from build123d import *

# Parameters (mm, degrees)
SKETCH_1_W                   = 50
SKETCH_1_H                   = 100
EXTRUDE_1_DEPTH              = 2
SKETCH_2_W                   = 3
SKETCH_2_H                   = 100
EXTRUDE_2_DEPTH              = 80
SKETCH_3_W                   = 2
SKETCH_3_H                   = 66.7
EXTRUDE_3_DEPTH              = 70
CUT_EXTRUDE_4_REACH          = 162.465
SKETCH_8_W                   = 2
SKETCH_8_H                   = 66.7
EXTRUDE_4_DEPTH              = 70
CUT_EXTRUDE_5_REACH          = 140.25
HOLE_WIZARD_M3_1_D           = 2.5
HOLE_WIZARD_M3_1_DEPTH       = 2
HOLE_WIZARD_M3_1_CSINK_D     = 3.05
HOLE_WIZARD_M3_1_CSINK_ANGLE = 90
FILLET_1_R                   = 2
CUT_EXTRUDE_6_REACH          = 140.25
SKETCH_12_R                  = 11
CUT_EXTRUDE_7_REACH          = 162.465
SKETCH_13_R                  = 14.5
SKETCH_14_W                  = 2
SKETCH_14_H                  = 66.7
EXTRUDE_5_DEPTH              = 70
CUT_EXTRUDE_8_REACH          = 156.14
SKETCH_15_R                  = 5.1
CUT_EXTRUDE_9_DEPTH          = 155.140358116
CUT_EXTRUDE_9_DEPTH_BACK     = 155.140358116
SKETCH_19_W                  = 2
SKETCH_19_H                  = 66.7
CUT_EXTRUDE_10_DEPTH         = 119.844436134
FILLET_2_R                   = 2
HOLE_WIZARD_M3_3_D           = 2.5
HOLE_WIZARD_M3_3_CSINK_D     = 3.05
HOLE_WIZARD_M3_3_CSINK_ANGLE = 90
CUT_EXTRUDE_11_DEPTH         = 134.88427839
CUT_EXTRUDE_11_DEPTH_BACK    = 134.88427839


# Read off the part's stored shape, not the designer's step: M1.6 螺纹孔1, M1.6 螺纹孔2, M2.5 螺纹孔1
with BuildPart() as part:
    # 草图1 → 凸台-拉伸1 (new body)
    with BuildSketch(Plane(origin=(0, 0, 0), x_dir=(1, 0, 0), z_dir=(0, 1, 0))):
        Rectangle(SKETCH_1_W, SKETCH_1_H)
    extrude(amount=EXTRUDE_1_DEPTH)

    # 草图2 → 凸台-拉伸2 (add)
    with BuildSketch(Plane(origin=(0, 2, 0), x_dir=(1, 0, 0), z_dir=(0, 1, 0))):
        with Locations((-23.5, 0)):
            Rectangle(SKETCH_2_W, SKETCH_2_H)
    extrude(amount=EXTRUDE_2_DEPTH)

    # 草图3 → 凸台-拉伸3 (add)
    with BuildSketch(Plane.ZY.offset(25)):
        with Locations((-49, 48.65)):
            Rectangle(SKETCH_3_W, SKETCH_3_H)
    extrude(amount=EXTRUDE_3_DEPTH)

    # 草图4 → 切除-拉伸4 (cut, up to next)
    with BuildSketch(Plane(origin=(0, 0, -50), x_dir=(-1, 0, 0), z_dir=(0, 0, -1)), mode=Mode.PRIVATE) as cut_extrude_4_sk1:
        with BuildLine():
            Line((95, 82), (61.65, 82))
            ThreePointArc((61.65, 82), (85.232011153, 72.232011153), (95, 48.65))
            Line((95, 48.65), (95, 82))
        make_face()
    cut_extrude_4_tool1 = extrude(cut_extrude_4_sk1.sketch, amount=-CUT_EXTRUDE_4_REACH, mode=Mode.PRIVATE) & part.part
    # 草图4 → 切除-拉伸4 (cut, up to next)
    with BuildSketch(Plane(origin=(0, 0, -50), x_dir=(-1, 0, 0), z_dir=(0, 0, -1)), mode=Mode.PRIVATE) as cut_extrude_4_sk2:
        with BuildLine():
            ThreePointArc((95, 48.65), (85.232011153, 25.067988847), (61.65, 15.3))
            Line((61.65, 15.3), (95, 15.3))
            Line((95, 15.3), (95, 48.65))
        make_face()
    cut_extrude_4_tool2 = extrude(cut_extrude_4_sk2.sketch, amount=-CUT_EXTRUDE_4_REACH, mode=Mode.PRIVATE) & part.part
    add(cut_extrude_4_tool1.solids().sort_by_distance((-87.550679, 74.550679, -50))[0], mode=Mode.SUBTRACT)
    add(cut_extrude_4_tool2.solids().sort_by_distance((-87.550679, 22.749321, -50))[0], mode=Mode.SUBTRACT)

    # 草图8 → 凸台-拉伸4 (add)
    with BuildSketch(Plane.ZY.offset(25)):
        with Locations((7, 48.65)):
            Rectangle(SKETCH_8_W, SKETCH_8_H)
    extrude(amount=EXTRUDE_4_DEPTH)

    # 草图9 → 切除-拉伸5 (cut, up to next)
    with BuildSketch(Plane.XY.offset(8), mode=Mode.PRIVATE) as cut_extrude_5_sk1:
        with BuildLine():
            ThreePointArc((-95, 48.65), (-85.232011153, 72.232011153), (-61.65, 82))
            Line((-61.65, 82), (-95, 82))
            Line((-95, 82), (-95, 48.65))
        make_face()
    cut_extrude_5_tool1 = extrude(cut_extrude_5_sk1.sketch, amount=-CUT_EXTRUDE_5_REACH, mode=Mode.PRIVATE) & part.part
    # 草图9 → 切除-拉伸5 (cut, up to next)
    with BuildSketch(Plane.XY.offset(8), mode=Mode.PRIVATE) as cut_extrude_5_sk2:
        with BuildLine():
            ThreePointArc((-61.65, 15.3), (-85.232011153, 25.067988847), (-95, 48.65))
            Line((-95, 48.65), (-95, 15.3))
            Line((-95, 15.3), (-61.65, 15.3))
        make_face()
    cut_extrude_5_tool2 = extrude(cut_extrude_5_sk2.sketch, amount=-CUT_EXTRUDE_5_REACH, mode=Mode.PRIVATE) & part.part
    add(cut_extrude_5_tool1.solids().sort_by_distance((-87.550679, 74.550679, 8))[0], mode=Mode.SUBTRACT)
    add(cut_extrude_5_tool2.solids().sort_by_distance((-87.550679, 22.749321, 8))[0], mode=Mode.SUBTRACT)

    # M3 螺纹孔1
    with Locations(Plane.XY.offset(8)):
        with Locations((-78.970508076, 38.65), (-61.65, 68.65), (-44.329491924, 38.65)):
            CounterSinkHole(HOLE_WIZARD_M3_1_D / 2, HOLE_WIZARD_M3_1_CSINK_D / 2, depth=HOLE_WIZARD_M3_1_DEPTH, counter_sink_angle=HOLE_WIZARD_M3_1_CSINK_ANGLE)

    # 圆角1
    fillet_1_edges = [part.edges().sort_by_distance(p)[0] for p in [
        (-23.5, 82, 50),
        (25, 1, 50),
        (25, 1, -50),
    ]]
    fillet(fillet_1_edges, radius=FILLET_1_R)

    # 草图12 → 切除-拉伸6 (cut, up to next)
    with BuildSketch(Plane.XY.offset(8), mode=Mode.PRIVATE) as cut_extrude_6_sk1:
        with Locations((-61.65, 48.65)):
            Circle(SKETCH_12_R)
    cut_extrude_6_tool1 = extrude(cut_extrude_6_sk1.sketch, amount=-CUT_EXTRUDE_6_REACH, mode=Mode.PRIVATE) & part.part
    add(cut_extrude_6_tool1.solids().sort_by_distance((-61.65, 48.65, 8))[0], mode=Mode.SUBTRACT)

    # 草图13 → 切除-拉伸7 (cut, up to next)
    with BuildSketch(Plane(origin=(0, 0, -50), x_dir=(-1, 0, 0), z_dir=(0, 0, -1)), mode=Mode.PRIVATE) as cut_extrude_7_sk1:
        with Locations((61.65, 48.65)):
            Circle(SKETCH_13_R)
    cut_extrude_7_tool1 = extrude(cut_extrude_7_sk1.sketch, amount=-CUT_EXTRUDE_7_REACH, mode=Mode.PRIVATE) & part.part
    add(cut_extrude_7_tool1.solids().sort_by_distance((-61.65, 48.65, -50))[0], mode=Mode.SUBTRACT)

    # 草图14 → 凸台-拉伸5 (add)
    with BuildSketch(Plane.ZY.offset(25)):
        with Locations((-38.5, 48.65)):
            Rectangle(SKETCH_14_W, SKETCH_14_H)
    extrude(amount=EXTRUDE_5_DEPTH)

    # 草图15 → 切除-拉伸8 (cut, up to next)
    with BuildSketch(Plane(origin=(0, 0, -39.5), x_dir=(-1, 0, 0), z_dir=(0, 0, -1)), mode=Mode.PRIVATE) as cut_extrude_8_sk1:
        with Locations(Location((61.65, 48.65, 0), (0, 0, 90))):
            Circle(SKETCH_15_R)
    cut_extrude_8_tool1 = extrude(cut_extrude_8_sk1.sketch, amount=-CUT_EXTRUDE_8_REACH, mode=Mode.PRIVATE) & part.part
    add(cut_extrude_8_tool1.solids().sort_by_distance((-61.65, 48.65, -39.5))[0], mode=Mode.SUBTRACT)

    # 草图18 → 切除-拉伸9 (cut, two sides: drawn at the far end of the back side and taken through both)
    with BuildSketch(Plane(origin=(0, 0, -39.5), x_dir=(-1, 0, 0), z_dir=(0, 0, -1)).offset(-CUT_EXTRUDE_9_DEPTH_BACK)):
        with BuildLine():
            Line((95, 15.3), (95, 48.65))
            ThreePointArc((95, 48.65), (85.232011153, 25.067988847), (61.65, 15.3))
            Line((61.65, 15.3), (95, 15.3))
        make_face()
        with BuildLine():
            Line((95, 48.65), (95, 82))
            Line((95, 82), (61.65, 82))
            ThreePointArc((61.65, 82), (85.232011153, 72.232011153), (95, 48.65))
        make_face()
    extrude(amount=CUT_EXTRUDE_9_DEPTH + CUT_EXTRUDE_9_DEPTH_BACK, mode=Mode.SUBTRACT)

    # 草图19 → 切除-拉伸10 (cut, through all)
    with BuildSketch(Plane.ZY.offset(25)):
        with Locations((-49, 48.65)):
            Rectangle(SKETCH_19_W, SKETCH_19_H)
    extrude(amount=CUT_EXTRUDE_10_DEPTH, mode=Mode.SUBTRACT)

    # 圆角2
    fillet_2_edges = [part.edges().sort_by_distance(p)[0] for p in [
        (-23.5, 82, -50),
    ]]
    fillet(fillet_2_edges, radius=FILLET_2_R)

    # M3 螺纹孔3 (through all)
    with Locations(Plane(origin=(0, 2, 0), x_dir=(1, 0, 0), z_dir=(0, 1, 0))):
        with Locations((-2.7, 0), (21, 10), (21, -10)):
            CounterSinkHole(HOLE_WIZARD_M3_3_D / 2, HOLE_WIZARD_M3_3_CSINK_D / 2, counter_sink_angle=HOLE_WIZARD_M3_3_CSINK_ANGLE)

    # M1.6 螺纹孔1 outline → M1.6 螺纹孔1 (revolve, cut)
    with BuildSketch(Plane(origin=(10, 0, -28), x_dir=(1, 0, 0), z_dir=(0, 0, 1))):
        Polygon((0, 0), (0.625, 0), (0.625, 1.8), (0.825, 2), (0, 2), align=None)
    revolve(axis=Axis((10, 0, -28), (0, 1, 0)), mode=Mode.SUBTRACT)

    # Hole Wizard M1.6 _1 2 outline → Hole Wizard M1.6 _1 2 (revolve, cut)
    with BuildSketch(Plane(origin=(6.4, 0, -28), x_dir=(1, 0, 0), z_dir=(0, 0, 1))):
        Polygon((0, 0), (0.625, 0), (0.625, 1.8), (0.825, 2), (0, 2), align=None)
    revolve(axis=Axis((6.4, 0, -28), (0, 1, 0)), mode=Mode.SUBTRACT)

    # M1.6 螺纹孔2 outline → M1.6 螺纹孔2 (revolve, cut)
    with BuildSketch(Plane(origin=(10, 0, -22), x_dir=(1, 0, 0), z_dir=(0, 0, 1))):
        Polygon((0, 0), (0.625, 0), (0.625, 1.8), (0.825, 2), (0, 2), align=None)
    revolve(axis=Axis((10, 0, -22), (0, 1, 0)), mode=Mode.SUBTRACT)

    # Hole Wizard M1.6 _2 2 outline → Hole Wizard M1.6 _2 2 (revolve, cut)
    with BuildSketch(Plane(origin=(6.4, 0, -22), x_dir=(1, 0, 0), z_dir=(0, 0, 1))):
        Polygon((0, 0), (0.625, 0), (0.625, 1.8), (0.825, 2), (0, 2), align=None)
    revolve(axis=Axis((6.4, 0, -22), (0, 1, 0)), mode=Mode.SUBTRACT)

    # 草图28 → 切除-拉伸11 (cut, two sides: drawn at the far end of the back side and taken through both)
    with BuildSketch(Plane(origin=(0, 2, 0), x_dir=(1, 0, 0), z_dir=(0, 1, 0)).offset(-CUT_EXTRUDE_11_DEPTH_BACK)):
        Polygon((-25, 37.5), (-95, 37.5), (-95, 39.5), (-25, 39.5), (-25, 50), (25, 50), (25, -50), (-25, -50), align=None)
    extrude(amount=CUT_EXTRUDE_11_DEPTH + CUT_EXTRUDE_11_DEPTH_BACK, mode=Mode.SUBTRACT)

    # M2.5 螺纹孔1 outline → M2.5 螺纹孔1 (revolve, cut)
    with BuildSketch(Plane(origin=(-29, 19, 0), x_dir=(1, 0, 0), z_dir=(0, -1, 0))):
        Polygon((0, 6), (1.025, 6), (1.025, 7.75), (1.275, 8), (0, 8), align=None)
    revolve(axis=Axis((-29, 19, 0), (0, 0, 1)), mode=Mode.SUBTRACT)

    # Hole Wizard M2.5 _1 2 outline → Hole Wizard M2.5 _1 2 (revolve, cut)
    with BuildSketch(Plane(origin=(-29, 27, 0), x_dir=(1, 0, 0), z_dir=(0, -1, 0))):
        Polygon((0, 6), (1.025, 6), (1.025, 7.75), (1.275, 8), (0, 8), align=None)
    revolve(axis=Axis((-29, 27, 0), (0, 0, 1)), mode=Mode.SUBTRACT)


solid = part.part
Build history of the part. All positions in model axes, mm. Round coordinates to 2 decimals unless told otherwise and drop trailing zeros. Loops run counter-clockwise (first coordinate to the right, second up) from the corner with the lowest first, then second, coordinate; pieces in that order, holes last. Notation, with made-up numbers: (51, 18) -> (61, 18) arc R12 cw to (61, 26) -> close; hole circle Ø4 at (0.5, 71). An arc over 180 degrees is marked (long way). One line per item, written item: value. Start each with the question number.
Q1. Probe line 1 along Y through (x, z) = (-61.65, 7); line 2 along Y through (x, z) = (-29, 6.8) (3 decimals); line 3 along X through (y, z) = (38.65, 6.75). List the from-to ranges inside material, lowest first.
Q2. Cut at A-A on z = 6.95. Count the separate pieces of the cut face and the enclosed holes in it, plus the area to 3 significant figures.
Q3. Cut at B-B on y = 27. List the corners of the cut face in (x, z) (3 decimals).
Q4. Two-plate mould, pull along Y, no slides. Class faces 1 (the face through (-52, 56, 8)), 2 (the face through (-43, 15.3, 7)), 3 (the face through (-45.001, 39.704, 6.85)): released by +Y, released by -Y, zero draft, split by the parting line, or undercut.
Q5. Cut at C-C on x = -68.5. List the corners of the cut face in (y, z), plus the area to 3 significant figures.
Computed:
1. line 1: 15.3 to 37.65, 59.65 to 67.4, 69.9 to 82
1. line 2: 15.3 to 17.975, 20.025 to 25.975, 28.025 to 82
1. line 3: -93.47 to -80.22, -77.72 to -66.23, -57.07 to -45.58, -43.08 to -25
2. separate pieces: 1
2. enclosed holes: 6
2. area: 3,790 mm²
3. outline: (-87.017, 6) -> (-30.025, 6) -> (-30.025, 7.75) -> (-30.275, 8) -> (-87.017, 8) -> close; (-27.975, 6) -> (-25, 6) -> (-25, 8) -> (-27.725, 8) -> (-27.975, 7.75) -> close
4. face 1: zero draft
4. face 2: released by -Y
4. face 3: undercut
5. outline: (16.01, 6) -> (40.04, 6) -> (40.04, 8) -> (16.01, 8) -> close; (57.26, 6) -> (81.29, 6) -> (81.29, 8) -> (57.26, 8) -> close
5. area: 96.1 mm²
